Input: part model. Units: mm. Frame: model coordinates. Face numbers are marked on the shaded views. Coordinates: 2 decimals unless noted, no trailing zeros. Write each loop counter-clockwise with the first axis right and the second up, starting at its lowest first coordinate (ties: lowest second). Pieces come first, ordered by that corner, then holes. Notation, with made-up numbers: (55, 64.5) - (112, 64.5) arc R22 cw to (112, 93.5) - close; hole circle Ø9 at (-11.5, -8). An arc over 180 degrees is marked (long way). Put each result on its own line as item: value. Start each with the question number.
1. Pin query (flat end, axial travel): pin 1 (1 mm diameter, centred on x = -0.5, y = -1, fed in from -Z). Return the tip coordinate at first contact, or that it passes through.
2. Pull-direction query (X, two-part tool) for the marked faces 1, 2 and 3; classes: released by +X, released by -X, zero draft, split by the parting line, or undercut.
3. Cut plane D-D, the plane y = 1.25. Return loops of the section in (x, z).
4. Cut plane C-C, the plane x = 0. Return loops of the section in (y, z), and give its area (4 significant figures).
5. Cut plane A-A, the plane y = 2. Return loops of the section in (x, z).
6. Line query: line 1 (X direction, y = -0.75, z = -0.2); line 2 (X direction, y = 1.5, z = -0.15); line 3 (Y direction, x = 2.5, z = -0.45). Output: solid intervals per line, ascending.
7. Cut plane B-B, the plane z = -0.3. Return loops of the section in (x, y).
from build123d import *

# Parameters (mm, degrees)
BODY_DEPTH = 0.6


with BuildPart() as part:
    # BodySke → Body (new body)
    with BuildSketch(Plane.XY):
        with BuildLine():
            Line((2.265769468, -1.056545654), (2.265769468, -2.224261502))
            ThreePointArc((2.265769468, -2.224261502), (2.522551556, -2.590803434), (2.95475915, -2.474671505))
            ThreePointArc((2.95475915, -2.474671505), (0, 3.854166667), (-2.95475915, -2.474671505))
            ThreePointArc((-2.95475915, -2.474671505), (-2.522551556, -2.590803434), (-2.265769468, -2.224261502))
            Line((-2.265769468, -2.224261502), (-2.265769468, -1.056545654))
            ThreePointArc((-2.265769468, -1.056545654), (-2.384292377, -0.751764499), (-2.462019383, -0.434120444))
            ThreePointArc((-2.462019383, -0.434120444), (-2.736711011, -0.311110876), (-2.82786799, -0.024270764))
            ThreePointArc((-2.82786799, -0.024270764), (0, 2.5), (2.82786799, -0.024270764))
            ThreePointArc((2.82786799, -0.024270764), (2.736711011, -0.311110876), (2.462019383, -0.434120444))
            ThreePointArc((2.462019383, -0.434120444), (2.384292377, -0.751764499), (2.265769468, -1.056545654))
        make_face()
    extrude(amount=-BODY_DEPTH)


solid = part.part
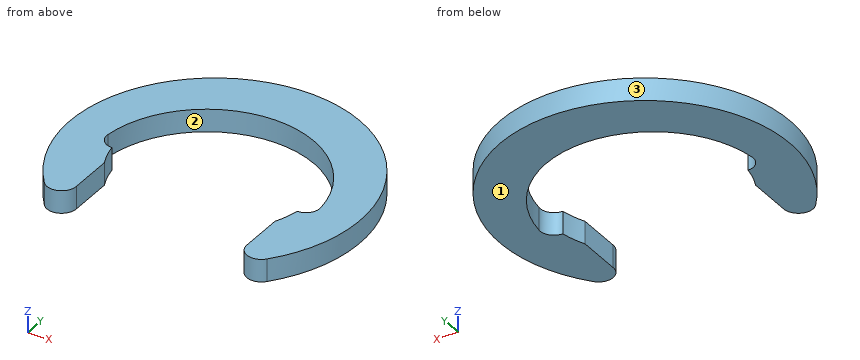
Report:
1. pin 1: passes through
2. face 1: zero draft
2. face 2: undercut
2. face 3: split by the parting line
3. outline: (-3.65, -0.6) - (-2.36, -0.6) - (-2.36, 0) - (-3.65, 0) - close; (2.36, -0.6) - (3.65, -0.6) - (3.65, 0) - (2.36, 0) - close
4. outline: (2.5, -0.6) - (3.85, -0.6) - (3.85, 0) - (2.5, 0) - close
4. area: 0.8125 mm^2
5. outline: (-3.29, -0.6) - (-1.61, -0.6) - (-1.61, 0) - (-3.29, 0) - close; (1.61, -0.6) - (3.29, -0.6) - (3.29, 0) - (1.61, 0) - close
6. line 1: x = -3.78 to -2.38, 2.38 to 3.78
6. line 2: x = -3.55 to -2.17, 2.17 to 3.55
6. line 3: y = -2.58 to -0.43, 1.01 to 2.93
7. outline: (-2.95, -2.47) arc R0.39 ccw to (-2.27, -2.22) - (-2.27, -1.06) arc R2.5 cw to (-2.46, -0.43) arc R0.37 cw to (-2.83, -0.02) arc R2.85 cw to (2.83, -0.02) arc R0.37 cw to (2.46, -0.43) arc R2.5 cw to (2.27, -1.06) - (2.27, -2.22) arc R0.39 ccw to (2.95, -2.47) arc R3.85 ccw (long way) to start
